Part model, mm, in its own coordinate system. A direction names the side the tool comes from. Round coordinates to 2 decimals unless told otherwise and drop trailing zeros. Order: outer loops, then holes, each group sorted by start corner. A loop starts at its lowest first (then second) coordinate and runs counter-clockwise, first axis right, second up. Notation, with made-up numbers: (-11, 68) -> (-6, 68) arc R24 ccw to (-6, 100) -> close; hole circle Ø9 at (39.25, 23.25). An arc over 180 degrees is marked (long way). Use CSV: the item, a comma, the result in double quotes.
```python
from build123d import *

# Parameters (mm, degrees)
SKETCH1_W                    = 42
SKETCH1_H                    = 1.23
BASE_FLANGE1_DEPTH           = 20
EDGE_FLANGE1_STRIP_W         = 6.3932
EDGE_FLANGE1_STRIP_H         = 1.23
EDGE_FLANGE1_STRIP_CUT_DEPTH = 42
EDGE_FLANGE1_DEPTH           = 42
SKETCH9_R                    = 1.984375
CUT_EXTRUDE1_DEPTH           = 30.516944286


# Sheet-metal steps are written as plain solids
with BuildPart() as part:
    # Sketch1 → Base-Flange1 (new body)
    with BuildSketch(Plane.XY):
        with Locations((0, -0.615)):
            Rectangle(SKETCH1_W, SKETCH1_H)
    extrude(amount=BASE_FLANGE1_DEPTH)

    # Edge-Flange1 strip (across the edge) → Edge-Flange1 strip cut (cut)
    with BuildSketch(Plane.ZY.offset(-21)):
        with Locations((-2.46, -0.615)):
            Rectangle(EDGE_FLANGE1_STRIP_W, EDGE_FLANGE1_STRIP_H)
    extrude(amount=EDGE_FLANGE1_STRIP_CUT_DEPTH, mode=Mode.SUBTRACT)

    # Edge-Flange1 section (across the edge) → Edge-Flange1 (add)
    with BuildSketch(Plane.ZY.offset(-21)):
        with BuildLine():
            Line((-1.23, 0.7366), (-1.23, 5.5))
            Line((-1.23, 5.5), (0, 5.5))
            Line((0, 5.5), (0, 0.7366))
            ThreePointArc((0, 0.7366), (0.215745145, 0.215745145), (0.7366, 0))
            Line((0.7366, 0), (0.7366, -1.23))
            ThreePointArc((0.7366, -1.23), (-0.653996196, -0.653996196), (-1.23, 0.7366))
        make_face()
    extrude(amount=EDGE_FLANGE1_DEPTH)

    # Sketch9 → Cut-Extrude1 (cut, through all)
    with BuildSketch(Plane(origin=(0, 0, 0), x_dir=(1, 0, 0), z_dir=(0, 1, 0))):
        with Locations(Location((-17, -10.7366, 0), (0, 0, 180))):
            Circle(SKETCH9_R)
    cut_extrude1 = extrude(amount=-CUT_EXTRUDE1_DEPTH, mode=Mode.SUBTRACT)

    # Mirror1: Cut-Extrude1 across plane
    add(cut_extrude1.mirror(Plane(origin=(0, 0, 0), x_dir=(0, 0, 1), z_dir=(1, 0, 0))), mode=Mode.SUBTRACT)


solid = part.part
```
(1) Cut at B-B, the plane z = 9.25. Give the cut face in (x, y), then the cut area to 3 significant figures.
Reply:
outline,"(-21, -1.23) -> (-18.31, -1.23) -> (-18.31, 0) -> (-21, 0) -> close; (-15.69, -1.23) -> (15.69, -1.23) -> (15.69, 0) -> (-15.69, 0) -> close; (18.31, -1.23) -> (21, -1.23) -> (21, 0) -> (18.31, 0) -> close"
area,"45.2 mm2"
(2) Which spindle directions (+Z, -Z, +X, -X, +Y, -Y) get a long thin tool onto all of the face, cutting with end or side? Do faces 4 (the face through (0, 3, 0)), 5 (the face through (21, -0.3, 7.9)). Say none if no direction does.
Reply:
face 4,"+Z, +X, -X, +Y"
face 5,"+Z, -Z, +X, +Y, -Y"
(3) Probe probe 1 along Z at (x, y) = (13, 3.5); probe 2 along Z at (x, y) = (-17, -0.5). List the from-to ranges inside material, lowest first. Write a range as [from, to].
Reply:
probe 1,"[-1.23, 0]"
probe 2,"[-0.79, 8.75], [12.72, 20]"
(4) Cut at C-C, the plane x = 13.5. Give the cut face in (y, z).
Reply:
outline,"(-1.23, 0.74) arc R1.97 ccw to (0.74, -1.23) -> (5.5, -1.23) -> (5.5, 0) -> (0.74, 0) arc R0.74 cw to (0, 0.74) -> (0, 20) -> (-1.23, 20) -> close"
(5) Cut at A-A, the plane x = -17. Give the cut face in (y, z), then the cut area to 3 significant figures.
Reply:
outline,"(-1.23, 0.74) arc R1.97 ccw to (0.74, -1.23) -> (5.5, -1.23) -> (5.5, 0) -> (0.74, 0) arc R0.74 cw to (0, 0.74) -> (0, 8.75) -> (-1.23, 8.75) -> close; (-1.23, 12.72) -> (0, 12.72) -> (0, 20) -> (-1.23, 20) -> close"
area,"27.3 mm2"
(6) Pull direction Z, two halves, no side cores. Call faces 1 (the face through (0, 3, -1.23)), 2 (the face through (0, -1.23, 10)), 3 (the face through (-17.92, -0.61, 8.98)): released by +Z, released by -Z, zero draft, split by the parting line, or undercut.
Reply:
face 1,"released by -Z"
face 2,"zero draft"
face 3,"undercut"
(7) Cut at D-D, the plane y = -0.5. Give the cut face in (x, z).
Reply:
outline,"(-21, -0.79) -> (21, -0.79) -> (21, 20) -> (-21, 20) -> close; hole circle Ø3.97 at (-17, 10.74); hole circle Ø3.97 at (17, 10.74)"
(8) Drop flat-ended pins along their axis: P1, Ø4, axis at y = 0.5, z = 10, coming from the +X side; P2, Ø1, axis at x = -1.5, y = 1, coming from the +Z side; P3, Ø12, axis at x = 12.5, z = 7.5, coming from the +Y side. Give the stop position or say it passes through.
Reply:
P1,"x = 21"
P2,"z = 0.04"
P3,"y = 0"
